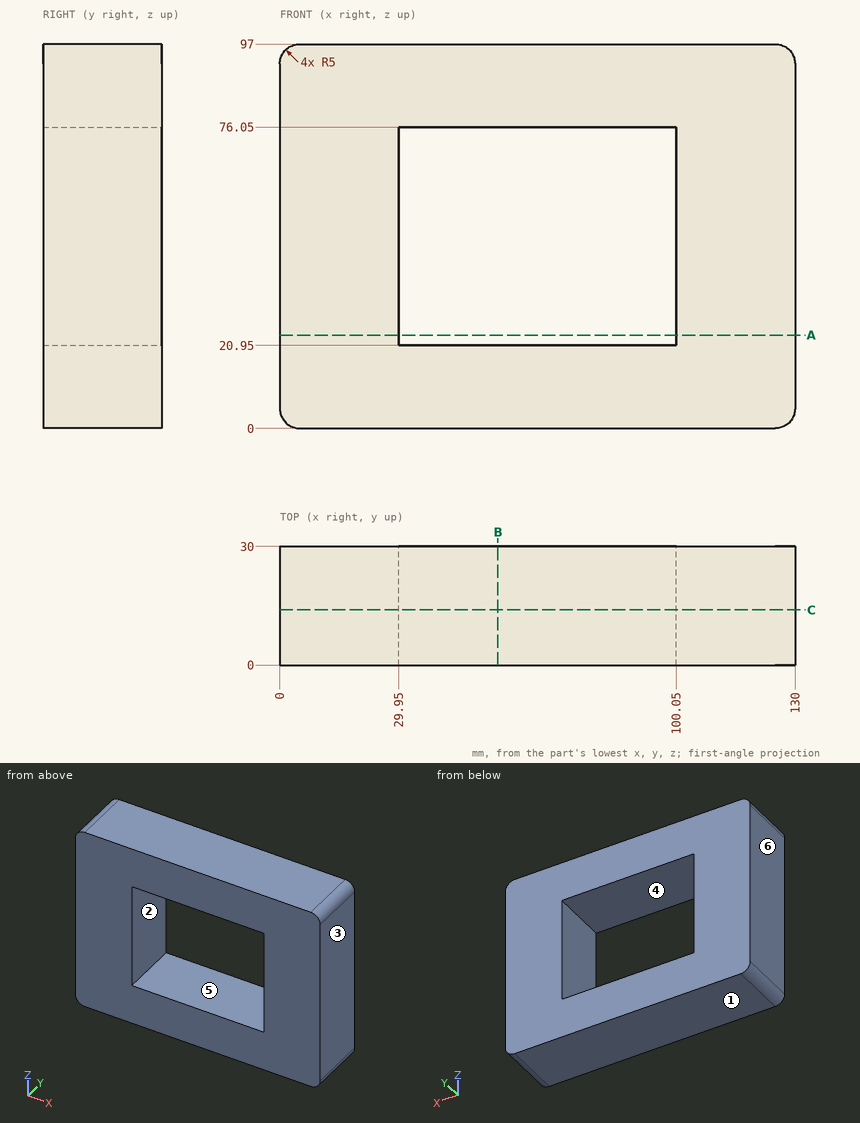
Source: three-view drawing plus pictorial views. Frame: mm from the lowest corner of the part. A direction names the side the tool comes from. Give positions to 0.01 mm unless a question says otherwise; leave off trailing zeros. Loops run counter-clockwise (first coordinate to the right, second up) from the corner with the lowest first, then second, coordinate; pieces in that order, holes last.
1) Reachability of the marked faces 1 and 2 from +Z, -Z, +X, -X, +Y, -Y: full face, straight path, thin tool, end or side. Return the list, or none.
A:
face 1: -Z, +X, -X, +Y, -Y
face 2: +Y, -Y
2) Section query B-B on x = 55. Return the cut outline in (y, z).
A:
outline: (0, 0) - (30, 0) - (30, 20.95) - (0, 20.95) - close; (0, 76.05) - (30, 76.05) - (30, 97) - (0, 97) - close
3) Section query C-C on y = 14. Return the cut outline in (x, z).
A:
outline: (0, 5) arc R5 ccw to (5, 0) - (125, 0) arc R5 ccw to (130, 5) - (130, 92) arc R5 ccw to (125, 97) - (5, 97) arc R5 ccw to (0, 92) - close; hole (29.95, 20.95) - (100.05, 20.95) - (100.05, 76.05) - (29.95, 76.05) - close
4) Section query A-A on z = 23.5. Return the cut outline in (x, y).
A:
outline: (0, 0) - (29.95, 0) - (29.95, 30) - (0, 30) - close; (100.05, 0) - (130, 0) - (130, 30) - (100.05, 30) - close
5) Mould query, pull axis X, two halves, no side actions, for the marked faces 3, 4, 5 and 6. Classes: released by +X, released by -X, zero draft, split by the parting line, or undercut.
A:
face 3: released by +X
face 4: undercut
face 5: undercut
face 6: released by -X
6) Contact query for a flat-ended pin moving along its axis: pin 1 (5 mm diameter, centred on y = 9, z = 48, fed in from -X). Output: stop coordinate, or through.
A:
pin 1: stops at x = 0
7) Line query: L1, parallel to Z at x = 62, y = 21; L2, parallel to X at y = 21.5, z = 25. Output: solid intervals per line, ascending.
A:
L1: z = 0 to 20.95, 76.05 to 97
L2: x = 0 to 29.95, 100.05 to 130
